```python
from build123d import *

# Parameters (mm, degrees)
SKETCH1_R                = 11.9
SKETCH1_R_2              = 9.9
BOSS_EXTRUDE3_DEPTH      = 15
SKETCH4_R                = 9.9
BOSS_EXTRUDE4_DEPTH      = 5.1
BOSS_EXTRUDE8_START      = -3
SKETCH12_R               = 19
SKETCH12_R_2             = 11.9
BOSS_EXTRUDE8_DEPTH      = 3
SKETCH14_R               = 1.755
CUT_EXTRUDE4_DEPTH       = 3
CUT_EXTRUDE5_DEPTH       = 25
CUT_EXTRUDE5_DEPTH_BACK  = 20
SKETCH15_W               = 38
SKETCH15_H               = 16.079993569
BOSS_EXTRUDE9_START      = -3
SKETCH16_R               = 9.9
BOSS_EXTRUDE9_DEPTH      = 3
BOSS_EXTRUDE10_START     = -3
SKETCH17_W               = 40
SKETCH17_H               = 40
SKETCH17_R               = 19
BOSS_EXTRUDE10_DEPTH     = 3
SKETCH20_W               = 60
SKETCH20_H               = 60
SKETCH20_W_2             = 40
SKETCH20_H_2             = 40
BOSS_EXTRUDE11_DEPTH     = 3
SKETCH21_R               = 1.755
CUT_EXTRUDE7_DEPTH       = 3
SKETCH23_W               = 60
SKETCH23_H               = 60
CUT_EXTRUDE9_DEPTH       = 3
BOSS_EXTRUDE12_START     = 3
SKETCH24_R               = 1.755
BOSS_EXTRUDE12_DEPTH     = 3
CUT_EXTRUDE10_DEPTH      = 16
CUT_EXTRUDE10_DEPTH_BACK = 42
SKETCH25_W               = 54.545590819
SKETCH25_H               = 6.512587561


with BuildPart() as part:
    # Sketch1 → Boss-Extrude3 (new body)
    with BuildSketch(Plane(origin=(0, 0, 0), x_dir=(1, 0, 0), z_dir=(0, 1, 0))):
        with Locations(Location((0, 0, 0), (0, 0, 270))):
            Circle(SKETCH1_R)
        with Locations(Location((0, 0, 0), (0, 0, 270))):
            Circle(SKETCH1_R_2, mode=Mode.SUBTRACT)
    extrude(amount=BOSS_EXTRUDE3_DEPTH)

    # Sketch4 → Boss-Extrude4 (add)
    with BuildSketch(Plane.XZ):
        with Locations(Location((0, 0, 0), (0, 0, 270))):
            Circle(SKETCH4_R)
    extrude(amount=-BOSS_EXTRUDE4_DEPTH)

    # Sketch7 → Cut-Revolve2 (revolve, cut)
    with BuildSketch(Plane(origin=(0, 0, 0), x_dir=(0, 0, -1), z_dir=(1, 0, 0))):
        with BuildLine():
            Line((0, 15), (0, -4.8))
            ThreePointArc((0, -4.8), (9.9, 5.1), (0, 15))
        make_face()
    revolve(axis=Axis((0, 15, 0), (0, -1, 0)), mode=Mode.SUBTRACT)

    # Sketch12 → Boss-Extrude8 (add)
    with BuildSketch(Plane(origin=(0, 15, 0), x_dir=(1, 0, 0), z_dir=(0, 1, 0)).offset(BOSS_EXTRUDE8_START)):
        with Locations(Location((0, 0, 0), (0, 0, 270))):
            Circle(SKETCH12_R)
        with Locations(Location((0, 0, 0), (0, 0, 270))):
            Circle(SKETCH12_R_2, mode=Mode.SUBTRACT)
    extrude(amount=BOSS_EXTRUDE8_DEPTH)

    # Sketch14 → Cut-Extrude4 (cut)
    with BuildSketch(Plane(origin=(0, 15, 0), x_dir=(1, 0, 0), z_dir=(0, 1, 0))):
        with Locations(Location((0, 15.15, 0), (0, 0, 270))):
            Circle(SKETCH14_R)
        with Locations(Location((-15.15, 0, 0), (0, 0, 270))):
            Circle(SKETCH14_R)
        with Locations(Location((0, -15.15, 0), (0, 0, 270))):
            Circle(SKETCH14_R)
        with Locations(Location((15.15, 0, 0), (0, 0, 270))):
            Circle(SKETCH14_R)
    extrude(amount=-CUT_EXTRUDE4_DEPTH, mode=Mode.SUBTRACT)

    # Sketch15 → Cut-Extrude5 (cut, two sides: drawn at the far end of the back side and taken through both)
    with BuildSketch(Plane(origin=(0, 0, 0), x_dir=(0, 0, -1), z_dir=(1, 0, 0)).offset(-CUT_EXTRUDE5_DEPTH_BACK)):
        with Locations((0, 3.960003216)):
            Rectangle(SKETCH15_W, SKETCH15_H)
    extrude(amount=CUT_EXTRUDE5_DEPTH + CUT_EXTRUDE5_DEPTH_BACK, mode=Mode.SUBTRACT)

    # Sketch16 → Boss-Extrude9 (add)
    with BuildSketch(Plane(origin=(0, 15, 0), x_dir=(1, 0, 0), z_dir=(0, 1, 0)).offset(BOSS_EXTRUDE9_START)):
        Circle(SKETCH16_R)
    extrude(amount=BOSS_EXTRUDE9_DEPTH)

    # Sketch17 → Boss-Extrude10 (add)
    with BuildSketch(Plane(origin=(0, 15, 0), x_dir=(1, 0, 0), z_dir=(0, 1, 0)).offset(BOSS_EXTRUDE10_START)):
        Rectangle(SKETCH17_W, SKETCH17_H)
        Circle(SKETCH17_R, mode=Mode.SUBTRACT)
    extrude(amount=BOSS_EXTRUDE10_DEPTH)

    # Sketch20 → Boss-Extrude11 (add)
    with BuildSketch(Plane(origin=(0, 15, 0), x_dir=(1, 0, 0), z_dir=(0, 1, 0))):
        Rectangle(SKETCH20_W, SKETCH20_H)
        Rectangle(SKETCH20_W_2, SKETCH20_H_2, mode=Mode.SUBTRACT)
    extrude(amount=-BOSS_EXTRUDE11_DEPTH)

    # Sketch21 → Cut-Extrude7 (cut)
    with BuildSketch(Plane(origin=(0, 15, 0), x_dir=(1, 0, 0), z_dir=(0, 1, 0))):
        with Locations(Location((-16.263455967, 16.263455967, 0), (0, 0, 270))):
            Circle(SKETCH21_R)
        with Locations(Location((-16.263455967, -16.263455967, 0), (0, 0, 270))):
            Circle(SKETCH21_R)
        with Locations(Location((16.263455967, 16.263455967, 0), (0, 0, 270))):
            Circle(SKETCH21_R)
        with Locations(Location((16.263455967, -16.263455967, 0), (0, 0, 270))):
            Circle(SKETCH21_R)
    extrude(amount=-CUT_EXTRUDE7_DEPTH, mode=Mode.SUBTRACT)

    # Sketch23 → Cut-Extrude9 (cut)
    with BuildSketch(Plane(origin=(0, 15, 0), x_dir=(1, 0, 0), z_dir=(0, 1, 0))):
        Rectangle(SKETCH23_W, SKETCH23_H)
        with BuildLine():
            Line((-20.263455967, -16.263455967), (-20.263455967, 16.263455967))
            ThreePointArc((-20.263455967, 16.263455967), (-19.091883092, 19.091883092), (-16.263455967, 20.263455967))
            Line((-16.263455967, 20.263455967), (16.263455967, 20.263455967))
            ThreePointArc((16.263455967, 20.263455967), (19.091883092, 19.091883092), (20.263455967, 16.263455967))
            Line((20.263455967, 16.263455967), (20.263455967, -16.263455967))
            ThreePointArc((20.263455967, -16.263455967), (19.091883092, -19.091883092), (16.263455967, -20.263455967))
            Line((16.263455967, -20.263455967), (-16.263455967, -20.263455967))
            ThreePointArc((-16.263455967, -20.263455967), (-19.091883092, -19.091883092), (-20.263455967, -16.263455967))
        make_face(mode=Mode.SUBTRACT)
    extrude(amount=-CUT_EXTRUDE9_DEPTH, mode=Mode.SUBTRACT)

    # Sketch24 → Boss-Extrude12 (add)
    with BuildSketch(Plane(origin=(0, 15, 0), x_dir=(1, 0, 0), z_dir=(0, 1, 0)).offset(BOSS_EXTRUDE12_START)):
        with BuildLine():
            Line((-19.091883092, 13.435028843), (-5.656854249, 0))
            Line((-5.656854249, 0), (-19.091883092, -13.435028843))
            ThreePointArc((-19.091883092, -13.435028843), (-19.091883092, -19.091883092), (-13.435028843, -19.091883092))
            Line((-13.435028843, -19.091883092), (0, -5.656854249))
            Line((0, -5.656854249), (13.435028843, -19.091883092))
            ThreePointArc((13.435028843, -19.091883092), (19.091883092, -19.091883092), (19.091883092, -13.435028843))
            Line((19.091883092, -13.435028843), (5.656854249, 0))
            Line((5.656854249, 0), (19.091883092, 13.435028843))
            ThreePointArc((19.091883092, 13.435028843), (19.091883092, 19.091883092), (13.435028843, 19.091883092))
            Line((13.435028843, 19.091883092), (0, 5.656854249))
            Line((0, 5.656854249), (-13.435028843, 19.091883092))
            ThreePointArc((-13.435028843, 19.091883092), (-19.091883092, 19.091883092), (-19.091883092, 13.435028843))
        make_face()
        with Locations(Location((-16.263455967, 16.263455967, 0), (0, 0, 270))):
            Circle(SKETCH24_R, mode=Mode.SUBTRACT)
        with Locations(Location((16.263455967, 16.263455967, 0), (0, 0, 270))):
            Circle(SKETCH24_R, mode=Mode.SUBTRACT)
        with Locations(Location((16.263455967, -16.263455967, 0), (0, 0, 270))):
            Circle(SKETCH24_R, mode=Mode.SUBTRACT)
        with Locations(Location((-16.263455967, -16.263455967, 0), (0, 0, 270))):
            Circle(SKETCH24_R, mode=Mode.SUBTRACT)
    extrude(amount=-BOSS_EXTRUDE12_DEPTH)

    # Sketch25 → Cut-Extrude10 (cut, two sides: drawn at the far end of the back side and taken through both)
    with BuildSketch(Plane.XY.offset(20.263455967).offset(-CUT_EXTRUDE10_DEPTH_BACK)):
        with Locations((4.016045733, 11.74370622)):
            Rectangle(SKETCH25_W, SKETCH25_H)
    extrude(amount=CUT_EXTRUDE10_DEPTH + CUT_EXTRUDE10_DEPTH_BACK, mode=Mode.SUBTRACT)


solid = part.part
```
Read the model definition and answer for the solid it produces. Units are mm, in the model's axes. A direction names the side the tool comes from. Coordinates: 2 decimals unless noted, no trailing zeros. Loops run counter-clockwise (first coordinate to the right, second up) from the corner with the lowest first, then second, coordinate; pieces in that order, holes last. Notation, with made-up numbers: (81.5, 29) -> (112.5, 29) arc R33 ccw to (112.5, 60) -> close; hole circle Ø7 at (10, 72). An arc over 180 degrees is marked (long way). Return JSON: item names as keys, results as strings.
Item 1: Find section C-C (y = 16.4). Determine the outline of the cut face in (x, z) (3 decimals).
Answers:
{"outline": "(-19.092, -13.435) arc R4 ccw to (-13.435, -19.092) -> (0, -5.657) -> (13.435, -19.092) arc R4 ccw to (19.092, -13.435) -> (5.657, 0) -> (19.092, 13.435) arc R4 ccw to (13.435, 19.092) -> (0, 5.657) -> (-13.435, 19.092) arc R4 ccw to (-19.092, 13.435) -> (-5.657, 0) -> close; hole circle Ø3.51 at (-16.263, -16.263); hole circle Ø3.51 at (-16.263, 16.263); hole circle Ø3.51 at (16.263, -16.263); hole circle Ø3.51 at (16.263, 16.263)"}
Item 2: Flat-ended cylindrical pins translate along their axes: P1, Ø1, axis at y = 15.5, z = 2, coming from the -X side; P2, Ø4.5, axis at x = -16.26, z = 16.26, coming from the -Y side. Find the tip coordinate at first contact, or state that the pin passes through.
Answers:
{"P1": "stops at x = -8.16", "P2": "stops at y = 15"}
Item 3: For a pull along Z with two mould halves and no side action, classify faces 5 (the flat face through (-6.812, 16.521, 12.468)), 6 (the flat face through (0, 15, 0)), 7 (the flat face through (12.28, 16.521, -6.623)) as +Z half, -Z half, draft (parallel to the pull), parting line (faces both ways), or undercut.
Answers:
{"face 5": "+Z half", "face 6": "draft", "face 7": "undercut"}
Item 4: Find section B-B (x = -11). Determine the outline of the cut face in (y, z), plus the area to 3 significant figures.
Answers:
{"outline": "(15, -16.66) -> (18, -16.66) -> (18, -5.34) -> (15, -5.34) -> close; (15, 5.34) -> (18, 5.34) -> (18, 16.66) -> (15, 16.66) -> close", "area": "67.9 mm2"}
Item 5: Find section D-D (z = 8). Determine the outline of the cut face in (x, y).
Answers:
{"outline": "(-13.66, 15) -> (-2.34, 15) -> (-2.34, 18) -> (-13.66, 18) -> close; (2.34, 15) -> (13.66, 15) -> (13.66, 18) -> (2.34, 18) -> close"}
Item 6: For faces 1 (the flat face through (12.468, 16.521, 6.812)), 2 (the flat face through (-12.468, 16.521, -6.812)), 3 (the flat face through (6.623, 16.521, 12.28)), 4 (the flat face through (6.812, 16.521, -12.468)), determine the directions among +Z, -Z, +X, -X, +Y, -Y from which every point of the face is accessible in a straight line to the end or side of a thin tool.
Answers:
{"face 1": "+X, +Y, -Y", "face 2": "-X, +Y, -Y", "face 3": "+Z, +Y, -Y", "face 4": "-Z, +Y, -Y"}
Item 7: Find section A-A (z = 15). Determine the outline of the cut face in (x, y).
Answers:
{"outline": "(-20.06, 15) -> (-17.48, 15) -> (-17.48, 18) -> (-20.06, 18) -> close; (-15.05, 15) -> (-9.34, 15) -> (-9.34, 18) -> (-15.05, 18) -> close; (9.34, 15) -> (15.05, 15) -> (15.05, 18) -> (9.34, 18) -> close; (17.48, 15) -> (20.06, 15) -> (20.06, 18) -> (17.48, 18) -> close"}
Item 8: Find the intervals of material crossed by probe 1 along X at (y, z) = (17.35, -17); probe 2 along Z at (x, y) = (12.5, 17.95); probe 3 along X at (y, z) = (17.3, -6), in increasing order.
Answers:
{"probe 1": "x = -20.2 to -17.86, -14.67 to -11.34, 11.34 to 14.67, 17.86 to 20.2", "probe 2": "z = -18.16 to -6.84, 6.84 to 18.16", "probe 3": "x = -11.66 to -0.34, 0.34 to 11.66"}
